Work out the finished part from the listing and answer in its coordinate system (mm). Round coordinates to 2 decimals unless told otherwise and drop trailing zeros. Order: outer loops, then holes, each group sorted by start corner. A loop starts at its lowest first (then second) coordinate and runs counter-clockwise, first axis right, second up. Notation, with made-up numbers: (-7, 39) -> (46, 39) arc R14 ccw to (46, 59) -> close; hole circle Ø1 at (62.25, 15). An arc over 180 degrees is marked (long way). Use one line per item in the form item = value.
```python
from build123d import *

# Parameters (mm, degrees)
F0_W         = 30
F0_H         = 30
F1_DEPTH     = 15
F2_R         = 5
F3_DEPTH     = 30.001
F4_R         = 5
F5_DEPTH     = 30.001
F6_R         = 5
F7_DEPTH     = 30.001
F8_R         = 5
F9_T1_DEPTH  = 20
F9_S5_W      = 5
F9_S5_H      = 5
F9_T6_DEPTH  = 5
F9_S11_W     = 5
F9_S11_H     = 5
F9_T12_DEPTH = 5


# Not quite as in the source:
# - a fillet or chamfer that OpenCascade refuses, or shapes differently, is made with other operations: its cross-section is extruded or revolved along the edge and cut away or added


with BuildPart() as f1:
    # F0 (on Top) → F1 (new body, symmetric)
    with BuildSketch(Plane.XY):
        Rectangle(F0_W, F0_H)
    extrude(amount=F1_DEPTH, both=True)

    # F2 (on face) → F3 (cut, through all)
    with BuildSketch(Plane.XY.offset(15)):
        Circle(F2_R)
    extrude(amount=-F3_DEPTH, mode=Mode.SUBTRACT)

    # F4 (on face) → F5 (cut, through all)
    with BuildSketch(Plane.YZ.offset(15)):
        Circle(F4_R)
    extrude(amount=-F5_DEPTH, mode=Mode.SUBTRACT)

    # F6 (on face) → F7 (cut, through all)
    with BuildSketch(Plane.XZ.offset(15)):
        Circle(F6_R)
    extrude(amount=-F7_DEPTH, mode=Mode.SUBTRACT)

    # F8
    f8_edges = [f1.edges().sort_by_distance(p)[0] for p in [
        (15, 0, 15),
        (0, 15, 15),
        (0, -15, 15),
        (-15, 0, 15),
        (-15, 15, 0),
        (15, -15, 0),
        (0, -15, -15),
        (-15, 0, -15),
        (15, 15, 0),
        (15, 0, -15),
        (-15, -15, 0),
    ]]
    fillet(f8_edges, radius=F8_R)

    # F9: fillet of radius 5 on 1 edges, made by hand

    # F9_s2 → F9_t1 (cut)
    with BuildSketch(Plane.YZ.offset(-10)):
        with BuildLine():
            ThreePointArc((15, -10), (13.5355339059, -13.5355339059), (10, -15))
            Line((10, -15), (15, -15))
            Line((15, -15), (15, -10))
        make_face()
    extrude(amount=F9_T1_DEPTH, mode=Mode.SUBTRACT)


with BuildPart() as f9_tool4:
    # F9_s5 → F9_t6 (new body)
    with BuildSketch(Plane.XZ.offset(-10)):
        with Locations((12.5, -12.5)):
            Rectangle(F9_S5_W, F9_S5_H)
    extrude(amount=-F9_T6_DEPTH)

    # F9_s7 → F9_t8 (revolve, cut)
    with BuildSketch(Plane(origin=(10, 10, -10), x_dir=(-0.7071067812, 0, 0.7071067812), z_dir=(-0.7071067812, 0, -0.7071067812))):
        with BuildLine():
            ThreePointArc((0, -5), (5, 0), (0, 5))
            Line((0, 5), (0, -5))
        make_face()
    revolve(axis=Axis((10, 10, -10), (0, 1, 0)), mode=Mode.SUBTRACT)


with BuildPart() as f1_1:
    add(f1.part)

    # F9_t3: cut F9_tool4
    add(f9_tool4.part, mode=Mode.SUBTRACT)


with BuildPart() as f9_tool10:
    # F9_s11 → F9_t12 (new body)
    with BuildSketch(Plane.XZ.offset(-10)):
        with Locations((-12.5, -12.5)):
            Rectangle(F9_S11_W, F9_S11_H)
    extrude(amount=-F9_T12_DEPTH)

    # F9_s13 → F9_t14 (revolve, cut)
    with BuildSketch(Plane(origin=(-10, 10, -10), x_dir=(0.7071067812, 0, 0.7071067812), z_dir=(-0.7071067812, 0, 0.7071067812))):
        with BuildLine():
            ThreePointArc((0, -5), (5, 0), (0, 5))
            Line((0, 5), (0, -5))
        make_face()
    revolve(axis=Axis((-10, 10, -10), (0, 1, 0)), mode=Mode.SUBTRACT)


with BuildPart() as f1_2:
    add(f1_1.part)

    # F9_t9: cut F9_tool10
    add(f9_tool10.part, mode=Mode.SUBTRACT)


solid = f1_2.part
```
Item 1: The part is cut by section B-B, the plane x = -4. Give the vertices of the cut face in (y, z), and give its area (3 significant figures).
Findings:
outline = (-15, -10) arc R5 ccw to (-10, -15) -> (-3, -15) -> (-3, -4) arc R5 cw to (-4, -3) -> (-15, -3) -> close; (-15, 3) -> (-4, 3) arc R5 cw to (-3, 4) -> (-3, 15) -> (-10, 15) arc R5 ccw to (-15, 10) -> close; (3, -15) -> (10, -15) arc R5 ccw to (15, -10) -> (15, -3) -> (4, -3) arc R5 cw to (3, -4) -> close; (3, 4) arc R5 cw to (4, 3) -> (15, 3) -> (15, 10) arc R5 ccw to (10, 15) -> (3, 15) -> close
area = 552 mm^2
Item 2: The part is cut by section D-D, the plane x = -9. Give the vertices of the cut face in (y, z), and give its area (3 significant figures).
Findings:
outline = (-15, -10) arc R5 ccw to (-10, -15) -> (10, -15) arc R5 ccw to (15, -10) -> (15, 10) arc R5 ccw to (10, 15) -> (-10, 15) arc R5 ccw to (-15, 10) -> close; hole circle Ø10 at (0, 0)
area = 800 mm^2
Item 3: Consider line 1 along Y through (x, z) = (0, 9.5); line 2 along Z through (x, y) = (0.25, 9); line 3 along X through (y, z) = (-7.25, 0.5). Determine where each line is inside the solid, lowest interval first.
Findings:
line_1 = -15 to -5, 5 to 15
line_2 = -15 to -4.99, 4.99 to 15
line_3 = -15 to -4.97, 4.97 to 15
Item 4: The part is cut by section A-A, the plane y = 0. Give the vertices of the cut face in (x, z), and give its area (3 significant figures).
Findings:
outline = (-15, -10) arc R5 ccw to (-10, -15) -> (-5, -15) -> (-5, -5) -> (-15, -5) -> close; (-15, 5) -> (-5, 5) -> (-5, 15) -> (-10, 15) arc R5 ccw to (-15, 10) -> close; (5, -15) -> (10, -15) arc R5 ccw to (15, -10) -> (15, -5) -> (5, -5) -> close; (5, 5) -> (15, 5) -> (15, 10) arc R5 ccw to (10, 15) -> (5, 15) -> close
area = 379 mm^2
Item 5: A flat-ended cylindrical pin translates along its axis: P1, Ø16, axis at y = 0, z = 0, coming from the +X side. Find the tip coordinate at first contact, or state that the pin passes through.
Findings:
P1 = 15
Item 6: Determine the mould class of faces 1 (the flat face through (-15, -5, 2)), 2 (the cylindrical face through (0, -14, -13)), 3 (the cylindrical face through (-5, 9, 0)), 4 (the cylindrical face through (-4, -9, 3)) for opening direction Z: released by +Z, released by -Z, zero draft, split by the parting line, or undercut.
Findings:
face_1 = zero draft
face_2 = released by -Z
face_3 = undercut
face_4 = undercut
